The listing builds one solid part. Answer for the finished solid, in the listing's coordinates (mm). A direction names the side the tool comes from. Round coordinates to 2 decimals unless told otherwise and drop trailing zeros. Order: outer loops, then holes, each group sorted by start corner. A loop starts at its lowest first (then second) coordinate and runs counter-clockwise, first axis right, second up. Notation, with made-up numbers: M 44.5,60.5 L 82.5,60.5 A18 ccw 82.5,65.5 Z; hole C -15,11.25 d7. An arc over 180 degrees is marked long. Write item = value, one per line. Start each with the question number.
(1) Straight lines are drawn through the part: probe 1 along Y at (x, z) = (0, 1.45); probe 2 along Z at (x, y) = (0.35, 23); probe 3 along X at (y, z) = (20.25, 0.6) (3 decimals). For each, find the intervals that lie inside material, in ascending order. Write a range as from..to.
(2) Which of the six approach directions +Z, -Z, +X, -X, +Y, -Y give full straight-line access (tool end or side, diameter ignored) to faces 1 (the face through (-0.26, 16.83, 1.25)), 2 (the face through (0, 30, 0.5))?
(3) Each of these flat-tipped pins is pushed along its axis until it touches: pin 1 (1.6 mm diameter, centred on x = 0, y = 18, fed in from -Z) (1 decimal); pin 2 (1.5 mm diameter, centred on x = -0.5, y = 21.5, fed in from +Z). Where does it stop, or does it pass through?
(4) For a pull along X with two mould halves and no side action, classify faces 3 (the face through (-0.13, 18.99, 1.25)), 4 (the face through (1.4, 18, 0.5)), 5 (the face through (0, 20, 1)), 6 (the face through (-0.217, 17.024, 0.493)) as released by +X, released by -X, zero draft, split by the parting line, or undercut.
(5) A cutting plane is placed at B-B, the plane y = 4.25. Determine the outline of the cut face in (x, z), and give its area (3 significant figures).
from build123d import *

# Parameters (mm, degrees)
ESBO_O1_R                = 1
RESSALTO_EXTRUS_O1_DEPTH = 1
ESBO_O3_R                = 1.2
ESBO_O3_R_2              = 0.999056936
RESSALTO_EXTRUS_O2_DEPTH = 0.5


with BuildPart() as part:
    # Esboço1 → Ressalto-extrusão1 (new body)
    with BuildSketch(Plane.XY):
        with BuildLine():
            Line((0, 30), (1, 30))
            Line((1, 30), (0.641479632, 19.244388959))
            ThreePointArc((0.641479632, 19.244388959), (1.39922287, 17.953359238), (0.557188515, 16.715655436))
            Line((0.557188515, 16.715655436), (0, 0))
            Line((0, 0), (-0.557188515, 16.715655436))
            ThreePointArc((-0.557188515, 16.715655436), (-1.39922287, 17.953359238), (-0.641479632, 19.244388959))
            Line((-0.641479632, 19.244388959), (-1, 30))
            Line((-1, 30), (0, 30))
        make_face()
        with Locations((0, 18)):
            Circle(ESBO_O1_R, mode=Mode.SUBTRACT)
    extrude(amount=RESSALTO_EXTRUS_O1_DEPTH)

    # Esboço3 → Ressalto-extrusão2 (add)
    with BuildSketch(Plane.XY.offset(1)):
        with Locations((0, 18)):
            Circle(ESBO_O3_R)
        with Locations((0, 18)):
            Circle(ESBO_O3_R_2, mode=Mode.SUBTRACT)
    extrude(amount=RESSALTO_EXTRUS_O2_DEPTH)


solid = part.part
Reported:
q1.probe_1 = 16.8..17, 19..19.2
q1.probe_2 = 0..1
q1.probe_3 = -0.675..0.675
q2.face_1 = +Z
q2.face_2 = +Z, -Z, +X, -X, +Y
q3.pin_1 = through
q3.pin_2 = 1
q4.face_3 = undercut
q4.face_4 = released by +X
q4.face_5 = zero draft
q4.face_6 = undercut
q5.outline = M -0.14,0 L 0.14,0 L 0.14,1 L -0.14,1 Z
q5.area = 0.283 mm²
